from build123d import *

# Parameters (mm, degrees)
BASEHEAD_DEPTH = 35


with BuildPart() as part:
    # BaseHeadSke → BaseHead (new body)
    with BuildSketch(Plane(origin=(0, 0, 0), x_dir=(0, 0, -1), z_dir=(1, 0, 0))):
        Polygon((0, 49.074772881), (-42.5, 24.537386441), (-42.5, -24.537386441), (0, -49.074772881), (42.5, -24.537386441), (42.5, 24.537386441), align=None)
    extrude(amount=BASEHEAD_DEPTH)

    # HeadChamferSke → HeadChamfer (revolve, cut)
    with BuildSketch(Plane.XY):
        Polygon((0, 49.074772881), (0, 42.5), (3.795946893, 49.074772881), align=None)
    revolve(axis=Axis((0, 0, 0), (1, 0, 0)), mode=Mode.SUBTRACT)

    # BodySke → BaseBody (revolve)
    with BuildSketch(Plane.XY, mode=Mode.PRIVATE) as basebody_sk:
        Polygon((0, 0), (0, 28), (391.9855, 28), (395, 24.9855), (395, 0), align=None)
    revolve(basebody_sk.sketch.rotate(Axis((0, 0, 0), (1, 0, 0)), 90), axis=Axis((0, 0, 0), (1, 0, 0)))


solid = part.part
For this review, take the finished solid that the model builds, in its own axes (mm). A direction names the side the tool comes from. Round coordinates to 2 decimals unless told otherwise and drop trailing zeros. Order: outer loops, then holes, each group sorted by start corner. A loop starts at its lowest first (then second) coordinate and runs counter-clockwise, first axis right, second up. Notation, with made-up numbers: M -16,71.5 L 27,71.5 A19 cw 27,96.5 Z; hole C 13,65.25 d6. An arc over 180 degrees is marked long. Use a Markdown table: item, result. Add a question column.
Item 1: Insertion check: pin 1 (6 mm diameter, centred on x = 136.5, y = -16.5, fed in from -Z); pin 2 (12 mm diameter, centred on x = 54, z = 16.5, fed in from -Y); pin 3 (3 mm diameter, centred on x = 252.5, z = -11, fed in from +Y). Each pin has a flat end and moves straight along its axis. Give the tip position at first contact, or say it passes through.
Item 2: Tool access review of faces 1 (the conical face through (0.92, 21.96, -38.24)), 2 (the cylindrical face through (215.99, 24.84, 12.92)): name each direction out of +Z, -Z, +X, -X, +Y, -Y from which nothing blocks a thin tool from reaching the whole face with its end or side.
Item 3: To check wall thickness, follow line 1 along Z through (x, y) = (367, 1); line 2 along X through (y, z) = (33, 9); line 3 along Y through (x, z) = (254, 0). State the ranges of each line that lie inside material, in increasing order.
Item 4: Add section A-A, the plane x = 310.5. Give the boundary of the cut face in (y, z).
Item 5: Mouldability with a two-part tool opening along X and no side actions: class faces 3 (the flat face through (17.255, 36.634, -21.547)), 4 (the flat face through (35, -21, 19)), 5 (the conical face through (0.923, -22.142, -38.136)) as released by +X, released by -X, zero draft, split by the parting line, or undercut.
Geometry results:
| question | item | result |
|---|---|---|
| 1 | pin 1 | stops at z = -24.53 |
| 1 | pin 2 | stops at y = -25.96 |
| 1 | pin 3 | stops at y = 26.34 |
| 2 | face 1 | -Z, -X, +Y |
| 2 | face 2 | +X |
| 3 | line 1 | z = -27.98 to 27.98 |
| 3 | line 2 | x = 0 to 35 |
| 3 | line 3 | y = -28 to 28 |
| 4 | outline | C 0,0 d56 |
| 5 | face 3 | zero draft |
| 5 | face 4 | released by +X |
| 5 | face 5 | released by -X |
